Here's how the part is built. I have some questions about the finished solid (model axes, mm). Face numbers are marked on the shaded views. Give positions to 0.01 mm unless a question says otherwise; leave off trailing zeros. Loops run counter-clockwise (first coordinate to the right, second up) from the corner with the lowest first, then second, coordinate; pieces in that order, holes last. Notation, with made-up numbers: (-39, 71) - (-22, 71) arc R15 ccw to (-22, 84) - close; hole circle Ø10 at (18, 80). An arc over 180 degrees is marked (long way). Use one line per item in the form item = value.
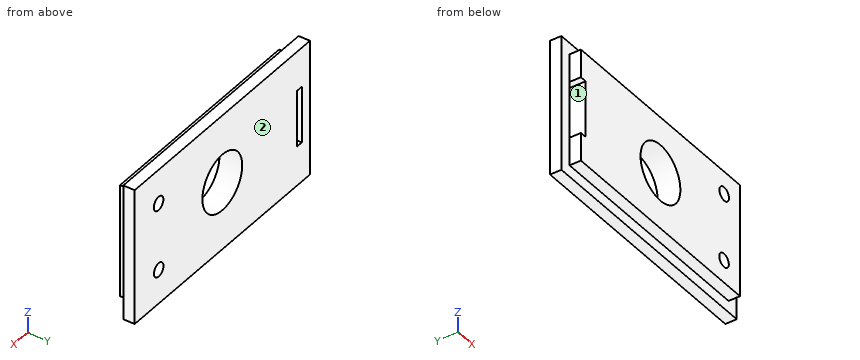
from build123d import *

# Parameters (mm, degrees)
SKETCH1_W           = 110
SKETCH1_H           = 60
BOSS_EXTRUDE1_DEPTH = 5
SKETCH2_W           = 99.8
SKETCH2_H           = 49.8
BOSS_EXTRUDE2_DEPTH = 5
SKETCH3_W           = 3
SKETCH3_H           = 25
CUT_EXTRUDE2_DEPTH  = 10
SKETCH5_R           = 3
CUT_EXTRUDE3_DEPTH  = 10
SKETCH6_R           = 12.5
CUT_EXTRUDE4_DEPTH  = 10


with BuildPart() as part:
    # Sketch1 → Boss-Extrude1 (new body)
    with BuildSketch(Plane(origin=(0, 0, 0), x_dir=(1, 0, 0), z_dir=(0, 1, 0))):
        Rectangle(SKETCH1_W, SKETCH1_H)
    extrude(amount=BOSS_EXTRUDE1_DEPTH)

    # Sketch2 → Boss-Extrude2 (add)
    with BuildSketch(Plane.XZ):
        Rectangle(SKETCH2_W, SKETCH2_H)
    extrude(amount=BOSS_EXTRUDE2_DEPTH)

    # Sketch3 → Cut-Extrude2 (cut)
    with BuildSketch(Plane.XZ.offset(5)):
        with Locations((-48.4, 0)):
            Rectangle(SKETCH3_W, SKETCH3_H)
    extrude(amount=-CUT_EXTRUDE2_DEPTH, mode=Mode.SUBTRACT)

    # Sketch5 → Cut-Extrude3 (cut)
    with BuildSketch(Plane.XZ.offset(5)):
        with Locations(Location((39.9, -14.9, 0), (0, 0, 270))):
            Circle(SKETCH5_R)
        with Locations(Location((40, 14.9, 0), (0, 0, 270))):
            Circle(SKETCH5_R)
    extrude(amount=-CUT_EXTRUDE3_DEPTH, mode=Mode.SUBTRACT)

    # Sketch6 → Cut-Extrude4 (cut)
    with BuildSketch(Plane(origin=(0, 5, 0), x_dir=(1, 0, 0), z_dir=(0, 1, 0))):
        with Locations(Location((0, 0, 0), (0, 0, 270))):
            Circle(SKETCH6_R)
    extrude(amount=-CUT_EXTRUDE4_DEPTH, mode=Mode.SUBTRACT)


solid = part.part
(1) If we section it at C-C (y = -1.25): List the corners of the cut face in (x, z) for me.
Geometry says:
outline = (-49.9, -24.9) - (49.9, -24.9) - (49.9, 24.9) - (-49.9, 24.9) - (-49.9, 12.5) - (-46.9, 12.5) - (-46.9, -12.5) - (-49.9, -12.5) - close; hole circle Ø25 at (0, 0); hole circle Ø6 at (39.9, -14.9); hole circle Ø6 at (40, 14.9)
(2) For P1, Ø4, axis at y = -3.5, z = 19, coming from the -X side; P2, Ø2.5, axis at y = -3.5, z = -4.5, coming from the +X side; P3, Ø1.5, axis at x = -12, y = -3.5, coming from the -Z side, each with a flat end and sliding along its axis, tell me the tip position at first contact or that it passes through.
Geometry says:
P1 = -49.9
P2 = 49.9
P3 = -24.9
(3) If we section it at A-A (x = 0): List the corners of the cut face in (y, z) for me, plus the area to 3 significant figures.
Geometry says:
outline = (-5, -24.9) - (0, -24.9) - (0, -30) - (5, -30) - (5, -12.5) - (-5, -12.5) - close; (-5, 12.5) - (5, 12.5) - (5, 30) - (0, 30) - (0, 24.9) - (-5, 24.9) - close
area = 299 mm²
(4) If we section it at B-B (z = -14.9): List the corners of the cut face in (x, y) for me, plus the area to 3 significant figures.
Geometry says:
outline = (-55, 0) - (-49.9, 0) - (-49.9, -5) - (36.9, -5) - (36.9, 5) - (-55, 5) - close; (42.9, -5) - (49.9, -5) - (49.9, 0) - (55, 0) - (55, 5) - (42.9, 5) - close
area = 989 mm²
(5) If we section it at D-D (z = 0): List the corners of the cut face in (x, y) for me, plus the area to 3 significant figures.
Geometry says:
outline = (-55, 0) - (-49.9, 0) - (-49.9, 5) - (-55, 5) - close; (-46.9, -5) - (-12.5, -5) - (-12.5, 5) - (-46.9, 5) - close; (12.5, -5) - (49.9, -5) - (49.9, 0) - (55, 0) - (55, 5) - (12.5, 5) - close
area = 769 mm²
(6) If I drill on probe 1 along X at (y, z) = (-0.75, 14.9); probe 2 along X at (y, z) = (2.75, 14.9); probe 3 along Z at (x, y) = (-49.5, -2.25), over which ranges is the centre line in solid material (lowest first)?
Geometry says:
probe_1 = -49.9 to 37, 43 to 49.9
probe_2 = -55 to 37, 43 to 55
probe_3 = -24.9 to -12.5, 12.5 to 24.9
(7) Thinking about a two-plate mould opening in X: for the marked faces 1 and 2, which applies, pulls with the +X half, pulls with the -X half, needs draft (parallel to the pull), parting line crosses it, or undercut?
Geometry says:
face_1 = undercut
face_2 = needs draft
